Design review of the part built by this model. Coordinates are the model's own, in mm. Face numbers are marked on the shaded views. A direction names the side the tool comes from. Round coordinates to 2 decimals unless told otherwise and drop trailing zeros. Order: outer loops, then holes, each group sorted by start corner. A loop starts at its lowest first (then second) coordinate and runs counter-clockwise, first axis right, second up. Notation, with made-up numbers: (25.5, -21) - (41.5, -21) arc R12 cw to (41.5, -14) - close; hole circle Ø2 at (79, 33.5). An arc over 180 degrees is marked (long way). Write item = value, one per line.
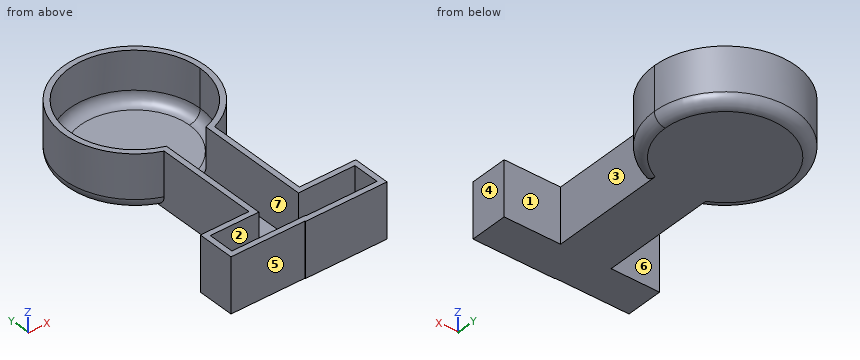
from build123d import *

# Parameters (mm, degrees)
F1_DEPTH = 25.4
F2_T     = -2.54
F3_R     = 5.08


with BuildPart() as f1:
    # F0 (on Top) → F1 (new body)
    with BuildSketch(Plane.XY):
        with BuildLine():
            ThreePointArc((-26.2971203774, -13.5154537857), (-38.0627484992, -15.6835315492), (-49.828376621, -13.5154537857))
            Line((-49.828376621, -13.5154537857), (-49.828376621, -61.4348314703))
            Line((-49.828376621, -61.4348314703), (-38.0627484992, -61.4348314703))
            Line((-38.0627484992, -61.4348314703), (-26.2971203774, -61.4348314703))
            Line((-26.2971203774, -61.4348314703), (-26.2971203774, -13.5154537857))
        make_face()
        with BuildLine():
            Line((-26.2971203774, -13.5154537857), (-49.828376621, -13.5154537857))
            ThreePointArc((-49.828376621, -13.5154537857), (-38.0627484992, -15.6835315492), (-26.2971203774, -13.5154537857))
        make_face()
        with BuildLine():
            ThreePointArc((-5.0541155298, 17.3251014203), (-56.7870982901, 44.5090778663), (-49.828376621, -13.5154537857))
            Line((-49.828376621, -13.5154537857), (-26.2971203774, -13.5154537857))
            ThreePointArc((-26.2971203774, -13.5154537857), (-10.8787720532, -1.3992483706), (-5.0541155298, 17.3251014203))
        make_face()
        Polygon((-38.0627484992, -61.4348314703), (-49.828376621, -61.4348314703), (-72.4281072617, -61.4348314703), (-72.4281072617, -78.7463337183), (-38.0627484992, -78.7463337183), align=None)
        Polygon((0, -61.4348314703), (-26.2971203774, -61.4348314703), (-38.0627484992, -61.4348314703), (-38.0627484992, -78.7463337183), (-38.0627484992, -79.0289491415), (0, -79.0289491415), align=None)
    extrude(amount=F1_DEPTH)

    # F2
    f2_openings = [f1.faces().sort_by_distance(p)[0] for p in [
        (-37.626368, -12.314928, 25.4),
    ]]
    offset(amount=F2_T, openings=f2_openings, kind=Kind.INTERSECTION)

    # F3
    f3_edges = [f1.edges().sort_by_distance(p)[0] for p in [
        (-38.062748, 47.793734, 2.54),
        (-38.062748, 50.333734, 0),
    ]]
    fillet(f3_edges, radius=F3_R)


solid = f1.part
Item 1: For the marked faces 4, 5, 6 and 7, list the 3-axis set-ups (+Z, -Z, +X, -X, +Y, -Y) from which the entire face can be reached by the end or side of a thin tool; tool diameter is ignored.
Data:
face_4 = +Z, -Z, +X, +Y, -Y
face_5 = +Z, -Z, -X, -Y
face_6 = +Z, -Z, -X
face_7 = +Z
Item 2: Take a section at A-A, the plane z = 11.25. State the section outline as (x, y) points, and give its area (3 significant figures).
Data:
outline = (-72.43, -78.75) - (-38.06, -78.75) - (-38.06, -79.03) - (0, -79.03) - (0, -61.43) - (-26.3, -61.43) - (-26.3, -13.52) arc R33.01 ccw (long way) to (-49.83, -13.52) - (-49.83, -61.43) - (-72.43, -61.43) - close; hole (-69.89, -76.21) - (-35.52, -76.21) - (-35.52, -76.49) - (-2.54, -76.49) - (-2.54, -63.97) - (-28.84, -63.97) - (-28.84, -11.71) arc R30.47 ccw (long way) to (-47.29, -11.71) - (-47.29, -63.97) - (-69.89, -63.97) - close
area = 1,080 mm2
Item 3: For line 1 along X through (y, z) = (-30.5, 24.25); line 2 along Y through (x, z) = (-15, 4.75); line 3 along Y through (x, z) = (-57.5, 14.5), list the stretches that pass through material, from the lowest coordinate up. Write a range as [from, to].
Data:
line_1 = [-49.83, -47.29], [-28.84, -26.3]
line_2 = [-79.03, -76.49], [-63.97, -61.43], [-6.28, -1.2], [35.85, 40.93]
line_3 = [-78.75, -76.21], [-63.97, -61.43], [-9.35, -6.14], [40.79, 44]
Item 4: The part is to be moulded in two halves that separate along X. For the marked faces 1, 2 and 3, say which applies: +X half, -X half, draft (parallel to the pull), parting line (faces both ways), or undercut.
Data:
face_1 = draft
face_2 = undercut
face_3 = +X half
Item 5: Insertion check: P1, Ø11.5, axis at x = -66, z = 14.5, coming from the +Y side; P2, Ø10, axis at y = 24.5, z = 3, coming from the -X side; P3, Ø7, axis at x = -56.5, z = 16, coming from the -Y side; P4, Ø5, axis at x = -46, y = 30.5, coming from the -Z side. Each pin has a flat end and moves straight along its axis. Give the tip position at first contact, or say it passes through.
Data:
P1 = 41.76
P2 = -70.97
P3 = -78.75
P4 = 0
